```python
from build123d import *

# Parameters (mm, degrees)
BOSS_EXTRUDE1_DEPTH  = 50
M3_CLEARANCE_HOLE1_D = 3.6
CUT_EXTRUDE1_START   = -41
CUT_EXTRUDE1_DEPTH   = 41
CUT_EXTRUDE2_DEPTH   = 2
FILLET1_R            = 1


with BuildPart() as part:
    # Sketch1 → Boss-Extrude1 (new body)
    with BuildSketch(Plane(origin=(0, 0, 0), x_dir=(1, 0, 0), z_dir=(0, 1, 0))):
        with BuildLine():
            Line((29.584742398, 81.283411698), (27.532621538, 75.645255973))
            ThreePointArc((27.532621538, 75.645255973), (24.694417894, 76.618768751), (21.821905854, 77.485833704))
            ThreePointArc((21.821905854, 77.485833704), (0, 84.853606671), (-21.821905854, 77.485833704))
            ThreePointArc((-21.821905854, 77.485833704), (-24.694417894, 76.618768751), (-27.532621538, 75.645255973))
            Line((-27.532621538, 75.645255973), (-29.584742398, 81.283411698))
            ThreePointArc((-29.584742398, 81.283411698), (0, 86.5), (29.584742398, 81.283411698))
        make_face()
    extrude(amount=-BOSS_EXTRUDE1_DEPTH)

    # M3 Clearance Hole1 (through all)
    with Locations(Plane(origin=(0, 0, 0), x_dir=(1, 0, 0), z_dir=(0, 1, 0))):
        with Locations((-25.108934259, 79.635365387), (25.108934259, 79.635365387)):
            Hole(M3_CLEARANCE_HOLE1_D / 2)

    # Sketch4 → Cut-Extrude1 (cut)
    with BuildSketch(Plane.XZ.offset(50).offset(CUT_EXTRUDE1_START)):
        with BuildLine():
            Line((-27.532621538, -75.645255973), (-29.584742398, -81.283411698))
            ThreePointArc((-29.584742398, -81.283411698), (-25.316064331, -82.712434898), (-20.978824316, -83.917453073))
            Line((-20.978824316, -83.917453073), (-21.821905854, -77.485833704))
            ThreePointArc((-21.821905854, -77.485833704), (-24.694417894, -76.618768751), (-27.532621538, -75.645255973))
        make_face()
        with BuildLine():
            Line((27.532621538, -75.645255973), (29.584742398, -81.283411698))
            ThreePointArc((29.584742398, -81.283411698), (25.316064331, -82.712434898), (20.978824316, -83.917453073))
            Line((20.978824316, -83.917453073), (21.821905854, -77.485833704))
            ThreePointArc((21.821905854, -77.485833704), (24.694417894, -76.618768751), (27.532621538, -75.645255973))
        make_face()
    extrude(amount=CUT_EXTRUDE1_DEPTH, mode=Mode.SUBTRACT)

    # Sketch5 → Cut-Extrude2 (cut)
    with BuildSketch(Plane(origin=(0, -9, 0), x_dir=(-1, 0, 0), z_dir=(0, -1, 0))):
        Polygon((25.559170371, 76.200647431), (28.30860532, 78.30792232), (27.858369208, 81.742640277), (24.658698146, 83.070083344), (21.909263197, 80.962808455), (22.359499309, 77.528090498), align=None)
        Polygon((-28.30860532, 78.30792232), (-25.559170371, 76.200647431), (-22.359499309, 77.528090498), (-21.909263197, 80.962808455), (-24.658698146, 83.070083344), (-27.858369208, 81.742640277), align=None)
    extrude(amount=-CUT_EXTRUDE2_DEPTH, mode=Mode.SUBTRACT)

    # Fillet1
    fillet1_edges = [part.edges().sort_by_distance(p)[0] for p in [
        (27.532621538, -4.5, -75.645255973),
        (29.584742398, -4.5, -81.283411698),
        (-29.584742398, -4.5, -81.283411698),
        (-27.532621538, -4.5, -75.645255973),
    ]]
    fillet(fillet1_edges, radius=FILLET1_R)


solid = part.part
```
Source: CAD feature listing. Evaluate the final solid. Frame: model axes, mm. A direction names the side the tool comes from. Give positions to 0.01 mm unless a question says otherwise; leave off trailing zeros. Order: outer loops, then holes, each group sorted by start corner. A loop starts at its lowest first (then second) coordinate and runs counter-clockwise, first axis right, second up.
(1) Section query C-C (y = -37). Return the cut outline in (x, z), plus the area to 3 significant figures.
(2) Section query A-A (y = -5). Return the cut outline in (x, z).
(3) Contact query for flat-ended pins moving along their axis: P1, Ø1.1, axis at x = 22, z = -81, coming from the -Y side; P2, Ø5, axis at y = -10, z = -78.5, coming from the -X side; P3, Ø2, axis at x = -7.5, y = -38, coming from the +Z side; P4, Ø4, axis at x = 16.5, y = -27, coming from the +Z side. Output: stop coordinate, or through.
(4) Pull-direction query (X, two-part tool) for faces 1 (the face through (22.1, -9, -81.4)), 2 (the face through (-25.94, -3.55, -78.04)), 3 (the face through (-28.547, -4.437, -78.432)); classes: +X half, -X half, draft (parallel to the pull), parting line (faces both ways), or undercut.
(5) Section query B-B (x = 16). Return the cut outline in (y, z).
(6) Material intervals for line 1 along X through (y, z) = (-19, -78.5); line 2 along X through (y, z) = (-21.5, -80.5); line 3 along Y through (x, z) = (-22.5, -78.75), sorted ascending.
(7) Access query for faces 4 (the face through (24.257, -4.437, -76.758)), 5 (the face through (26.537, -3.549, -78.54)), 6 (the face through (-21.4, -29.2, -80.7)), 7 (the face through (22.138, -8.014, -79.221)), 8 (the face through (-28.44, -9, -78.69)). Directions: +Z, -Z, +X, -X, +Y, -Y. A direction counts if a zero-diameter tool reaches every point of the face in a straight line with its end or side. Return the directions, or none.
Outcome:
1. outline: (-21.82, -77.49) - (-20.98, -83.92) arc R86.5 ccw to (20.98, -83.92) - (21.82, -77.49) arc R36 cw to start
1. area: 129 mm2
2. outline: (-29.24, -80.34) arc R1 ccw to (-28.63, -81.62) arc R86.5 ccw to (28.63, -81.62) arc R1 ccw to (29.24, -80.34) - (27.87, -76.58) arc R1 ccw to (26.6, -75.98) arc R80.5 cw to (21.82, -77.49) arc R36 cw to (-21.82, -77.49) arc R80.5 cw to (-26.6, -75.98) arc R1 ccw to (-27.87, -76.58) - close; hole circle Ø3.6 at (-25.11, -79.64); hole circle Ø3.6 at (25.11, -79.64)
3. P1: stops at y = -9
3. P2: stops at x = -29.3
3. P3: stops at z = -83.84
3. P4: stops at z = -79.74
4. face 1: draft
4. face 2: undercut
4. face 3: -X half
5. outline: (-50, -85.01) - (0, -85.01) - (0, -81.1) - (-50, -81.1) - close
6. line 1: x = -21.69 to -20.42, 20.42 to 21.69
6. line 2: x = -21.43 to -17.16, 17.16 to 21.43
6. line 3: y = -7 to 0
7. face 4: +Z, +Y, -Y
7. face 5: +Y, -Y
7. face 6: -Z, -X, -Y
7. face 7: -Y
7. face 8: +Z, -Z, -X, -Y
